```python
from build123d import *

# Parameters (mm, degrees)
CROQUIS1_W              = 900
CROQUIS1_H              = 100
CROQUIS1_H_2            = 150
SALIENTE_EXTRUIR2_DEPTH = 25
CORTAR_EXTRUIR1_DEPTH   = 10
CROQUIS3_W              = 950
CROQUIS3_H              = 25
CORTAR_EXTRUIR2_DEPTH   = 750


with BuildPart() as part:
    # Croquis1 → Saliente-Extruir2 (new body)
    with BuildSketch(Plane(origin=(0, 0, 0), x_dir=(1, 0, 0), z_dir=(0, 1, 0))):
        Polygon((450, -475), (450, -575), (100, -575), (100, -600), (475, -600), (475, 600), (-475, 600), (-475, -600), (-100, -600), (-100, -575), (-450, -575), (-450, -475), align=None)
        with Locations((0, -325)):
            Rectangle(CROQUIS1_W, CROQUIS1_H, mode=Mode.SUBTRACT)
        with Locations((0, 50)):
            Rectangle(CROQUIS1_W, CROQUIS1_H_2, mode=Mode.SUBTRACT)
        with Locations((0, 350)):
            Rectangle(CROQUIS1_W, CROQUIS1_H_2, mode=Mode.SUBTRACT)
    extrude(amount=SALIENTE_EXTRUIR2_DEPTH)

    # Croquis2 → Cortar-Extruir1 (cut)
    with BuildSketch(Plane(origin=(-100, 0, 0), x_dir=(0, 0, -1), z_dir=(1, 0, 0))):
        with BuildLine():
            ThreePointArc((-583.75, 12.5), (-586.064937129, 15.964548247), (-590.151650429, 15.151650429))
            Line((-590.151650429, 15.151650429), (-584.848349571, 9.848349571))
            ThreePointArc((-584.848349571, 9.848349571), (-584.035451753, 11.064937129), (-583.75, 12.5))
        make_face()
        with BuildLine():
            Line((-584.848349571, 9.848349571), (-590.151650429, 15.151650429))
            ThreePointArc((-590.151650429, 15.151650429), (-590.151650429, 9.848349571), (-584.848349571, 9.848349571))
        make_face()
    extrude(amount=-CORTAR_EXTRUIR1_DEPTH, mode=Mode.SUBTRACT)

    # Croquis3 → Cortar-Extruir2 (cut)
    with BuildSketch(Plane(origin=(0, 0, -600), x_dir=(-1, 0, 0), z_dir=(0, 0, -1))):
        with Locations((0, 12.5)):
            Rectangle(CROQUIS3_W, CROQUIS3_H)
    extrude(amount=-CORTAR_EXTRUIR2_DEPTH, mode=Mode.SUBTRACT)


solid = part.part
```
Model file for the job. Use its own axes, mm. A direction names the side the tool comes from. Round coordinates to 2 decimals unless told otherwise and drop trailing zeros. Write each loop counter-clockwise with the first axis right and the second up, starting at its lowest first coordinate (ties: lowest second). Pieces come first, ordered by that corner, then holes. Notation, with made-up numbers: (-9, 51.5) -> (17, 51.5) arc R19 ccw to (17, 61.5) -> close; hole circle Ø5 at (43, 20.25). An arc over 180 degrees is marked (long way). Answer as CSV lines item,"result".
1. Slice it at A-A, the plane z = 361.5. List the corners of the cut face in (x, y).
Resolved:
outline,"(-475, 0) -> (-450, 0) -> (-450, 25) -> (-475, 25) -> close; (450, 0) -> (475, 0) -> (475, 25) -> (450, 25) -> close"
2. Mould opens along Z. For faces 4 (the face through (285, 12, 600)), 5 (the face through (-475, 12, 372)), 6 (the face through (-450, 12, 326)) say: +Z half, -Z half, draft (parallel to the pull), parting line (faces both ways), or undercut.
Resolved:
face 4,"+Z half"
face 5,"draft"
face 6,"undercut"
3. Slice it at C-C, the plane x = -17. List the corners of the cut face in (y, z), plus the area to 4 significant figures.
Resolved:
outline,"(0, 150) -> (25, 150) -> (25, 275) -> (0, 275) -> close; (0, 375) -> (25, 375) -> (25, 475) -> (0, 475) -> close"
area,"5,625 mm²"
4. Drill centre lines: line 1 (Z direction, x = -183, y = 3); line 2 (X direction, y = 4.25, z = 547); line 3 (Z direction, x = 86.5, y = 14). Where is each one in solid material? Low to high.
Resolved:
line 1,"150 to 275, 375 to 475, 575 to 600"
line 2,"-475 to -450, 450 to 475"
line 3,"150 to 275, 375 to 475"
5. Slice it at D-D, the plane x = -292. List the corners of the cut face in (y, z).
Resolved:
outline,"(0, 150) -> (25, 150) -> (25, 275) -> (0, 275) -> close; (0, 375) -> (25, 375) -> (25, 475) -> (0, 475) -> close; (0, 575) -> (25, 575) -> (25, 600) -> (0, 600) -> close"
6. Slice it at B-B, the plane y = 21. List the corners of the cut face in (x, z).
Resolved:
outline,"(-475, 150) -> (475, 150) -> (475, 600) -> (100, 600) -> (100, 575) -> (450, 575) -> (450, 475) -> (-450, 475) -> (-450, 575) -> (-100, 575) -> (-100, 600) -> (-475, 600) -> close; hole (-450, 275) -> (450, 275) -> (450, 375) -> (-450, 375) -> close"
7. Pin check, flat tip, straight feed: pin 1 Ø7.5 at (x, y) = (59.5, 14.5) entering from +Z. Stop position of the tip, or through.
Resolved:
pin 1,"z = 475"
8. Tool access for faces 1 (the face through (277, 12, 575)), 2 (the face through (475, 12, 378)), 3 (the face through (-100, 9.5, 590.5)): list every direction of +Z, -Z, +X, -X, +Y, -Y with a clear straight run to the whole face (end or side of a thin tool).
Resolved:
face 1,"+Y, -Y"
face 2,"+Z, -Z, +X, +Y, -Y"
face 3,"+Z, +Y, -Y"
